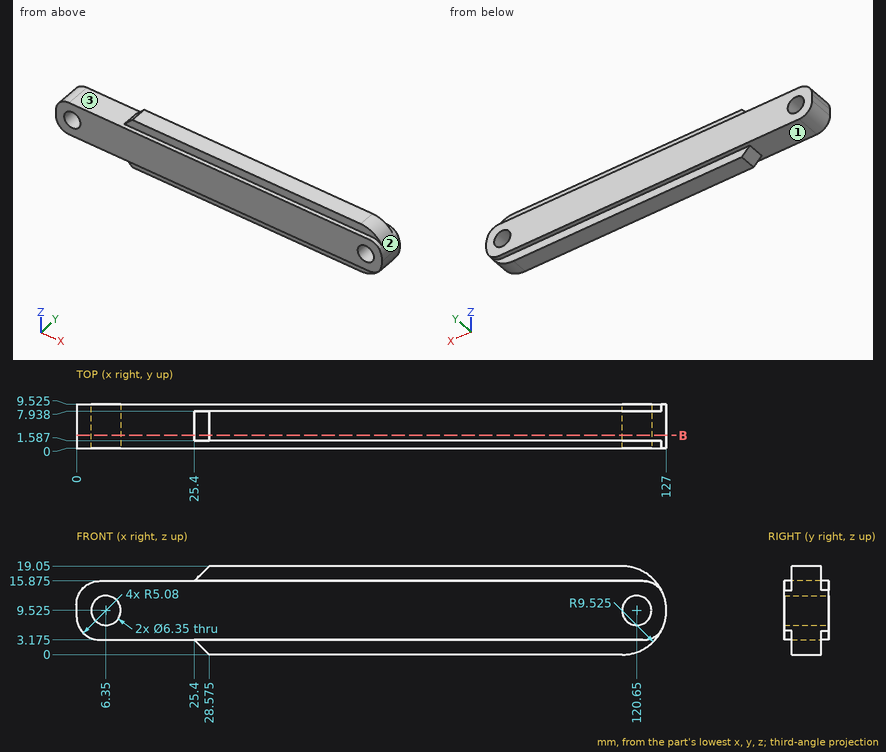
Here's the drawing with two shaded views (mm, measured from the low corner). I have some questions. A direction names the side the tool comes from. Coordinates: 2 decimals unless noted, no trailing zeros. Return JSON: item names as keys, results as strings. Group by question number.
Item 1: Imagine slicing it at B-B (y = 2.75). Give the number of separate pieces and of enclosed holes in the cut face, and give its area (3 significant figures).
Item 2: On a 3-axis mill with a long thin cutter (end or side, diameter ignored), from which of +Z, -Z, +X, -X, +Y, -Y can I reach the whole of each face in a straight line? I mean the marked faces 1, 2 and 3. Say none if no direction works.
Item 3: If I drill on L1, parallel to X at y = 4.75, z = 9.5 (1 decimal); L2, parallel to X at y = 5.5, z = 8.5 (1 decimal); L3, parallel to Y at x = 56, z = 2.5, over which ranges is the centre line in solid material (lowest first)? Write a range as from..to.
Item 4: I'm going to push flat-ended pins straight in: pin 1 Ø2 at (y, z) = (5, 8.5) entering from +X; pin 2 Ø5 at (y, z) = (1.5, 4) entering from +X; pin 3 Ø2 at (y, z) = (4, 15.5) entering from -X (1 decimal). Where does each tip first touch, or does it pass through?
Verdict:
{
 "1": {"separate pieces": "1", "enclosed holes": "2", "area": "2,130 mm^2"},
 "2": {"face 1": "-Z, -X", "face 2": "+Z, +X, +Y, -Y", "face 3": "+Z, -X"},
 "3": {"L1": "x = 0..3.2, 9.5..117.5, 123.8..127", "L2": "x = 0..3.3, 9.4..117.6, 123.7..126.9", "L3": "y = 1.59..7.94"},
 "4": {"pin 1": "stops at x = 127", "pin 2": "stops at x = 126.51", "pin 3": "stops at x = 1.6"}
}
